```python
from build123d import *

# Parameters (mm, degrees)
BOSS_EXTRUDE1_DEPTH = 1
BOSS_EXTRUDE2_DEPTH = 1
CUT_EXTRUDE1_DEPTH  = 208.84850252


with BuildPart() as part:
    # Sketch1 → Boss-Extrude1 (new body)
    with BuildSketch(Plane(origin=(0, 0, 0), x_dir=(1, 0, 0), z_dir=(0, 1, 0))):
        with BuildLine():
            Line((-141.421356237, 50), (-50, 50))
            Line((-50, 50), (-50, 141.421356237))
            ThreePointArc((-50, 141.421356237), (-106.066017178, 106.066017178), (-141.421356237, 50))
        make_face()
        with BuildLine():
            Line((-50, 30), (-50, 50))
            Line((-50, 50), (-141.421356237, 50))
            ThreePointArc((-141.421356237, 50), (-144.541706249, 40.096074055), (-146.969384567, 30))
            Line((-146.969384567, 30), (-50, 30))
        make_face()
        with BuildLine():
            Line((-50, 50), (-30, 50))
            Line((-30, 50), (-30, 146.969384567))
            ThreePointArc((-30, 146.969384567), (-40.096074055, 144.541706249), (-50, 141.421356237))
            Line((-50, 141.421356237), (-50, 50))
        make_face()
    extrude(amount=BOSS_EXTRUDE1_DEPTH)

    # Sketch2 → Boss-Extrude2 (add)
    with BuildSketch(Plane(origin=(0, 1, 0), x_dir=(-1, 0, 0), z_dir=(0, 1, 0))):
        with BuildLine():
            Line((50, -50), (141.421356237, -50))
            ThreePointArc((141.421356237, -50), (106.066017178, -106.066017178), (50, -141.421356237))
            Line((50, -141.421356237), (50, -50))
        make_face()
    extrude(amount=BOSS_EXTRUDE2_DEPTH)

    # Sketch3 → Cut-Extrude1 (cut, through all)
    with BuildSketch(Plane(origin=(0, 1, 0), x_dir=(1, 0, 0), z_dir=(0, 1, 0))):
        with BuildLine():
            Line((-141.421356237, 50), (-50, 50))
            Line((-50, 50), (-50, 30))
            Line((-50, 30), (-146.969384567, 30))
            ThreePointArc((-146.969384567, 30), (-144.541706249, 40.096074055), (-141.421356237, 50))
        make_face()
    extrude(amount=-CUT_EXTRUDE1_DEPTH, mode=Mode.SUBTRACT)


solid = part.part
```
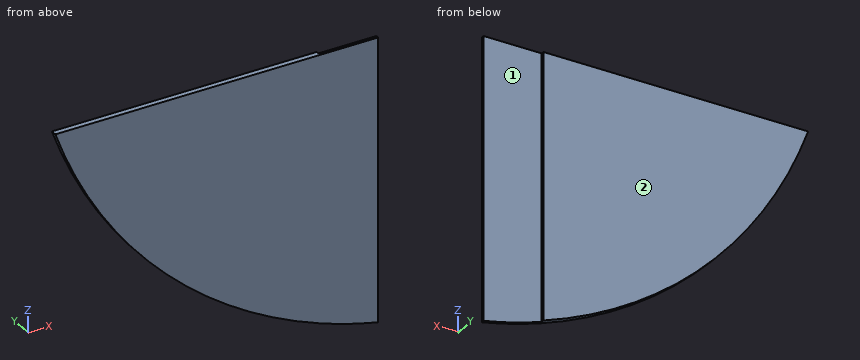
Work out the finished part from the listing and answer in its coordinate system (mm). Face numbers are marked on the shaded views. A direction names the side the tool comes from. Coordinates: 2 decimals unless noted, no trailing zeros. Order: outer loops, then holes, each group sorted by start corner. A loop starts at its lowest first (then second) coordinate and runs counter-clockwise, first axis right, second up. Notation, with made-up numbers: M 39,70.5 L 94,70.5 A22 cw 94,88.5 Z; hole C -6.5,63 d7. An arc over 180 degrees is marked long. Use CSV: the item, a comma, the result in double quotes.
1) Section C-C on z = -111 is taken. Write down the section's boundary in (x, y), plus the area to 3 significant figures.
Worked out:
outline,"M -100.89,0 L -30,0 L -30,1 L -50,1 L -50,2 L -100.89,2 Z"
area,"122 mm^2"
2) Section D-D on z = -69 is taken. Write down the section's boundary in (x, y).
Worked out:
outline,"M -133.19,0 L -30,0 L -30,1 L -50,1 L -50,2 L -133.19,2 Z"
3) Section B-B on x = -42 is taken. Write down the section's boundary in (y, z).
Worked out:
outline,"M 0,-144 L 1,-144 L 1,-50 L 0,-50 Z"
4) For the marked faces 1 and 2, determine the directions among +Z, -Z, +X, -X, +Y, -Y from which every point of the face is accessible in a straight line to the end or side of a thin tool.
Worked out:
face 1,"+Z, -Z, +X, +Y"
face 2,"+Z, -Z, +X, -X, +Y"
5) Flat-ended cylindrical pins translate along their axes: pin 1 Ø1 at (y, z) = (2, -101) entering from +X; pin 2 Ø16 at (x, z) = (-40.5, -111) entering from +Y. Find the tip coordinate at first contact, or state that the pin passes through.
Worked out:
pin 1,"stops at x = -50"
pin 2,"stops at y = 1"
6) Consider line 1 (Y direction, x = -36, z = -119.5); line 2 (X direction, y = 0.9, z = -118); line 3 (X direction, y = 1.3, z = -126). Determine where each line is inside the solid, lowest interval first. Write a range as [from, to].
Worked out:
line 1,"y = [0, 1]"
line 2,"x = [-92.61, -30]"
line 3,"x = [-81.39, -50]"
7) Section A-A on y = 0.35 is taken. Write down the section's boundary in (x, z), plus the area to 3 significant figures.
Worked out:
outline,"M -141.42,-50 A150 ccw -30,-146.97 L -30,-50 Z"
area,"7,340 mm^2"
